The drawing under review shows one solid part. Ordinate dimensions are in mm from its lowest x, y, z. A direction names the side the tool comes from. Coordinates: 2 decimals unless noted, no trailing zeros. Loops run counter-clockwise (first coordinate to the right, second up) from the corner with the lowest first, then second, coordinate; pieces in that order, holes last. Notation, with made-up numbers: M -33.75,82 L -24.75,82 A21 ccw -24.75,107 Z; hole C 78,-11 d1. An arc over 180 degrees is marked long. Return JSON: item names as keys, results as strings.
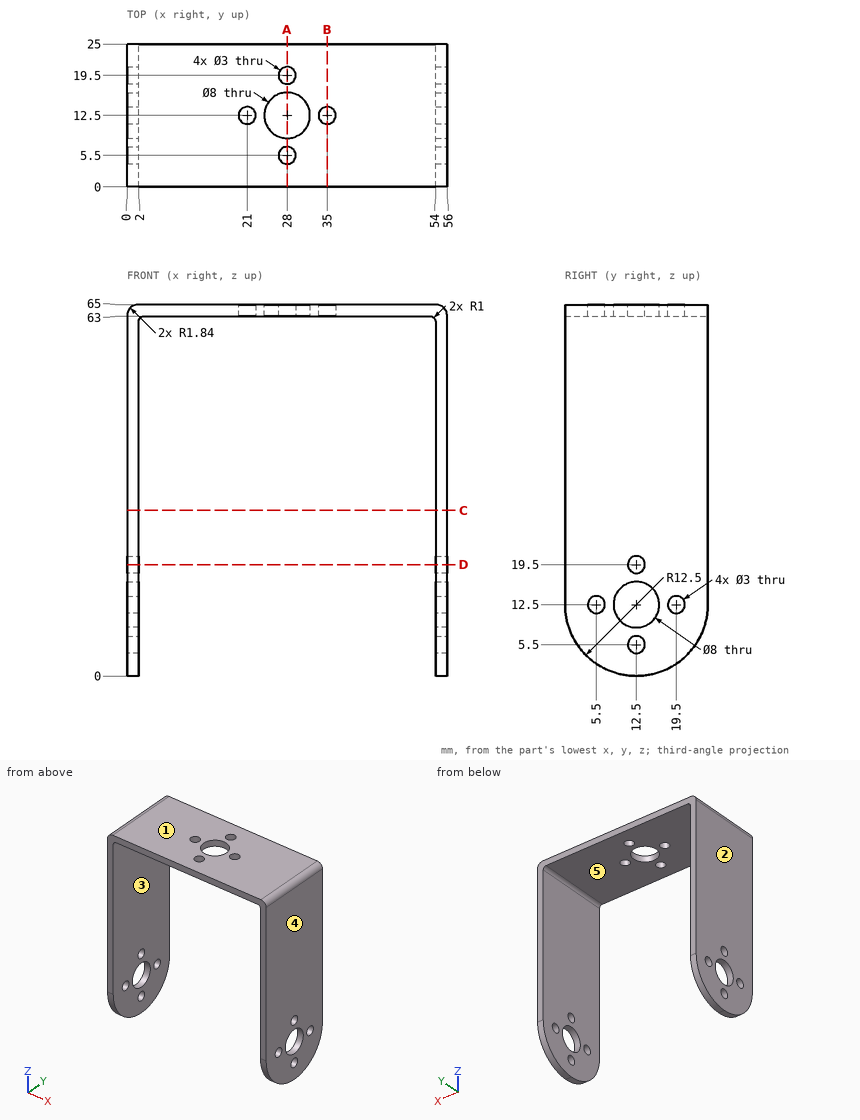
1. Add section A-A on x = 28. Give the boundary of the cut face in (y, z), plus the area to 3 significant figures.
Check values:
{"outline": "M 0,63 L 4,63 L 4,65 L 0,65 Z; M 7,63 L 8.5,63 L 8.5,65 L 7,65 Z; M 16.5,63 L 18,63 L 18,65 L 16.5,65 Z; M 21,63 L 25,63 L 25,65 L 21,65 Z", "area": "22.0 mm²"}
2. Insertion check: pin 1 Ø1.8 at (x, y) = (35, 12.5) entering from +Z; pin 2 Ø8 at (x, y) = (34.5, 12) entering from -Z. Each pin has a flat end and moves straight along its axis. Give the tip position at first contact, or say it passes through.
Check values:
{"pin 1": "through", "pin 2": "z = 63"}
3. Add section D-D on z = 19.5. Give the boundary of the cut face in (x, y), plus the area to 3 significant figures.
Check values:
{"outline": "M 0,0 L 2,0 L 2,11 L 0,11 Z; M 0,14 L 2,14 L 2,25 L 0,25 Z; M 54,0 L 56,0 L 56,11 L 54,11 Z; M 54,14 L 56,14 L 56,25 L 54,25 Z", "area": "88.0 mm²"}
4. Add section C-C on z = 29. Give the boundary of the cut face in (x, y).
Check values:
{"outline": "M 0,0 L 2,0 L 2,25 L 0,25 Z; M 54,0 L 56,0 L 56,25 L 54,25 Z"}
5. To check wall thickness, follow line 1 (Y direction, x = 55.3, z = 12.5); line 2 (X direction, y = 15.5, z = 9.5); line 3 (Y direction, x = 35, z = 64.15). State the ranges of each line that lie inside material, in increasing order.
Check values:
{"line 1": "0 to 4, 7 to 8.5, 16.5 to 18, 21 to 25", "line 2": "0 to 2, 54 to 56", "line 3": "0 to 11, 14 to 25"}
6. Add section B-B on x = 35. Give the boundary of the cut face in (y, z), plus the area to 3 significant figures.
Check values:
{"outline": "M 0,63 L 11,63 L 11,65 L 0,65 Z; M 14,63 L 25,63 L 25,65 L 14,65 Z", "area": "44.0 mm²"}
7. Machinability: for the marked faces 4 and 5, which of the approach directions +Z, -Z, +X, -X, +Y, -Y give a long, thin tool a straight path to every point of the face, cutting with its end or side? Answer none if there is none.
Check values:
{"face 4": "+Z, -Z, +X, +Y, -Y", "face 5": "-Z, +Y, -Y"}
8. The part is to be moulded in two halves that separate along X. For the marked faces 1, 2 and 3, say which applies: released by +X, released by -X, zero draft, split by the parting line, or undercut.
Check values:
{"face 1": "zero draft", "face 2": "released by -X", "face 3": "undercut"}
